Part model, mm, in its own coordinate system. A direction names the side the tool comes from. Coordinates: 2 decimals unless noted, no trailing zeros. Loops run counter-clockwise (first coordinate to the right, second up) from the corner with the lowest first, then second, coordinate; pieces in that order, holes last. Notation, with made-up numbers: M 29,-39 L 66,-39 A12 cw 66,-31 Z; hole C 19.25,58 d4. An arc over 180 degrees is marked long. Answer as CSV lines item,"result". Start each with the question number.
Autodesk Inventor part; units mm, degrees
ref_plane "YZ Plane" through (0, 0, 0) normal (1, 0, 0) x (0, 1, 0)
ref_plane "XZ Plane" through (0, 0, 0) normal (0, 1, 0) x (-1, 0, 0)
ref_plane "XY Plane" through (0, 0, 0) normal (0, 0, 1) x (1, 0, 0)
sketch "Sketch1" plane through (0, 0, 0) normal (0, 0, 1) x (1, 0, 0)
  line L0 (0, 0) -> (55, 0)
  line L1 (0, 0) -> (35, 0)
  line L2 (35, 3.8429) -> (35, 4.5)
  line L3 (29.0376, 3.7334) -> (0, 0)
  line L4 (41.7595, 2.9791) -> (55, 0)
  arc A0 (43.1851, 2.6584) -> (25.4094, 3.2669) centre (32.8243, -40.0614) ccw
  line L5 (-5.4039, 0) -> (70.1536, 0)
  line L6 (0, 0) -> (27.5, 0)
  line L7 (25.4094, 0) -> (29.1094, 0)
  line L8 (29.1094, 0) -> (29.1094, 2.5)
  line L9 (29.1094, 2.5) -> (25.4094, 2.5)
  line L10 (25.4094, 2.5) -> (25.4094, 0)
  dimension "d0" = 55
  dimension "d1" = 35
  dimension "d2" = 4.5
  dimension "d5" = 27.5
  dimension "d6" = 3.7
  dimension "d7" = 2.5
extrude "Extrusion1" add sketch "Sketch1" along normal blind 245 contours L3 A0 L4 L0 L8 L9 L10 | L10 L9 L8 L0
mirror "Mirror1" about plane through (0, 0, 0) normal (0, 1, 0) of "Extrusion1"
sketch "Sketch2" plane through (0, 0, 245) normal (0, 0, 1) x (1, 0, 0)
  line L0 (29.0376, 3.7334) -> (0, 0)
  line L1 (0, 0) -> (27.5, 0)
  line L2 (27.5, 0) -> (27.5, 3)
  line L3 (27.5, 3) -> (24.8907, 3)
  line L4 (24.8907, 3) -> (24.8907, -3.2002)
  line L5 (29.0376, -3.7334) -> (0, 0)
  line L6 (24.8907, 3) -> (30.3823, 3)
  line L7 (30.3823, 3) -> (30.3823, -3.2002)
  line L8 (30.3823, -3.2002) -> (24.8907, -3.2002)
  line L9 (24.8907, -3.2002) -> (24.8907, 3)
  dimension "d8" = 27.5
  dimension "d9" = 3
extrude "Extrusion2" add sketch "Sketch2" along normal blind 10 contours L4 L3 L2 L1 | L1 L2 L6 L7 L8 L4
ref_plane "Work Plane1" through (24.8907, -0.1, 245) normal (0, 1, 0) x (1, 0, 0)
sketch "Sketch3" plane through (24.8907, -0.1, 245) normal (0, 1, 0) x (1, 0, 0)
  line L0 (5.4916, -10) -> (-0.0004, -10)
  line L1 (-0.0004, -10) -> (-0.0004, -35.5)
  line L2 (-0.0004, -35.5) -> (5.4916, -35.5)
  line L3 (5.4916, -35.5) -> (5.4916, -10)
  circle A0 centre (2.7456, -35.5) radius 24
  circle A1 centre (2.7456, -35.5) radius 5.25
  point P0 (-24.8907, 245)
  dimension "d13" = 5.492
  dimension "d14" = 25.5
  dimension "d15" = 48
  dimension "d16" = 10.5
extrude "Extrusion3" add sketch "Sketch3" along normal blind 4 and the other way blind 4 contours A0 L1 A1 L3 | L3 A1 L1 A0
sketch "Sketch4" plane through (0, 0, 255) normal (0, 0, 1) x (1, 0, 0)
  line L0 (24.8907, -3.2002) -> (30.3823, -3.2002)
  line L1 (24.8907, 3) -> (24.8907, -3.2002)
  line L2 (30.3823, -3.2002) -> (24.8907, -3.2002)
  line L3 (24.8907, -3.2002) -> (24.8907, 3)
  line L4 (24.8907, 3) -> (30.3823, 3)
  line L5 (30.3823, 3) -> (30.3823, -3.2002)
  point P0 (0, 0)
extrude "Extrusion4" add sketch "Sketch4" along normal blind 15
properties part number "Ruder"
Q1. Flat gauge pins, fed straight in: P1, Ø1.9, axis at y = -1, z = 248, coming from the -X side; P2, Ø2, axis at x = 16.5, z = 187, coming from the +Y side; P3, Ø4.5, axis at x = 29, z = 249.5, coming from the -Y side. Where does each tip first touch, or does it go through?
Q2. Tool access for faces 4 (the face through (35.515, -3.814, 120.785)), 5 (the face through (48.47, -1.47, 120.78)), 6 (the face through (35.337, 3.825, 120.785)), 7 (the face through (30.382, 0, 251)), 8 (the face through (48.29, 1.51, 120.78)): list every direction of +Z, -Z, +X, -X, +Y, -Y with a clear straight run to the whole face (end or side of a thin tool).
Q3. Two-plate mould, pull along Z, no slides. Class faces 1 (the face through (27, 0, 0)), 2 (the face through (30.5, -0.2, 284.9)), 3 (the face through (14.722, 1.893, 120.785)): +Z half, -Z half, draft (parallel to the pull), parting line (faces both ways), or undercut.
Q4. Slice it at A-A, the plane x = 8. Write the cut outline in (y, z), and give its area (3 significant figures).
Q5. Wall check: L1, parallel to X at y = 0.75, z = 280.5; L2, parallel to Y at x = 33, z = 233.5; L3, parallel to Y at x = 42, z = 19. Give the ranges that are in metal, low to high.
Q6. Slice it at B-B, the plane z = 280.5. Write the cut outline in (x, y).
Q7. Slice it at C-C, the plane z = 174. Write the cut outline in (x, y), and give its area (3 significant figures).
Solved:
1,P1,"stops at x = 24.89"
1,P2,"stops at y = 2.25"
1,P3,"stops at y = -3.2"
2,face 4,"-Z, -Y"
2,face 5,"-Z, +X, -Y"
2,face 6,"-Z, +Y"
2,face 7,"+X, +Y, -Y"
2,face 8,"-Z, +X, +Y"
3,face 1,"-Z half"
3,face 2,"undercut"
3,face 3,"draft"
4,outline,"M -4.1,266.7 L 3.9,266.7 L 3.9,294.3 L -4.1,294.3 Z; M -1.03,0 L 1.03,0 L 1.03,245 L -1.03,245 Z"
4,area,"725 mm2"
5,L1,"x = 3.64 to 22.39, 32.89 to 51.64"
5,L2,"y = -3.9 to 3.9"
5,L3,"y = -2.92 to 2.92"
6,outline,"M 3.64,-4.1 L 22.39,-4.1 L 22.39,3.9 L 3.64,3.9 Z; M 32.89,-4.1 L 51.64,-4.1 L 51.64,3.9 L 32.89,3.9 Z"
7,outline,"M 0,0 L 29.04,-3.73 A43.96 ccw 41.76,-2.98 L 55,0 L 41.76,2.98 A43.96 ccw 29.04,3.73 Z"
7,area,"241 mm2"
